```python
from build123d import *

# Parameters (mm, degrees)
F0_W     = 12.5
F0_H     = 7
F1_DEPTH = 8
F2_DEPTH = 2.5


# Not quite as in the source:
# - a feature names something its author has since deleted; it is built from what else it names


with BuildPart() as f1:
    # F0 (on Top) → F1 (new body)
    with BuildSketch(Plane.XY):
        Polygon((-3.75, 44.5469365077), (-3.6919084378, 44.5469365077), (-3.6919084378, 71.5469365077), (-3.6919084378, 78.5469365077), (-8.75, 78.5469365077), (-8.75, 44.5469365077), align=None)
        Polygon((8.75, -44.5469365077), (8.75, 44.5469365077), (3.75, 44.5469365077), (-3.6919084378, 44.5469365077), (-3.75, 44.5469365077), (-8.75, 44.5469365077), (-8.75, -44.5469365077), align=None)
        with BuildLine():
            Line((-4.25, -2.5992627119), (4.25, -2.5992627119))
            Line((4.25, -2.5992627119), (4.25, -17.016687017))
            ThreePointArc((4.25, -17.016687017), (5.7282196187, -19.0992627119), (6.25, -21.5992627119))
            ThreePointArc((6.25, -21.5992627119), (5.7282196187, -24.0992627119), (4.25, -26.1818384069))
            Line((4.25, -26.1818384069), (4.25, -40.5992627119))
            Line((4.25, -40.5992627119), (-4.25, -40.5992627119))
            Line((-4.25, -40.5992627119), (-4.25, -26.1818384069))
            ThreePointArc((-4.25, -26.1818384069), (-6.25, -21.5992627119), (-4.25, -17.016687017))
            Line((-4.25, -17.016687017), (-4.25, -2.5992627119))
        make_face(mode=Mode.SUBTRACT)
        with Locations((2.5580915622, 75.0469365077)):
            Rectangle(F0_W, F0_H)
    extrude(amount=F1_DEPTH)

    # F0 (on Top) → F2 (join)
    with BuildSketch(Plane.XY):
        with BuildLine():
            Line((4.25, -40.5992627119), (4.25, -26.1818384069))
            ThreePointArc((4.25, -26.1818384069), (0, -27.8492627119), (-4.25, -26.1818384069))
            Line((-4.25, -26.1818384069), (-4.25, -40.5992627119))
            Line((-4.25, -40.5992627119), (4.25, -40.5992627119))
        make_face()
        with BuildLine():
            Line((4.25, -26.1818384069), (4.25, -17.016687017))
            ThreePointArc((4.25, -17.016687017), (0, -15.3492627119), (-4.25, -17.016687017))
            Line((-4.25, -17.016687017), (-4.25, -26.1818384069))
            ThreePointArc((-4.25, -26.1818384069), (0, -27.8492627119), (4.25, -26.1818384069))
        make_face()
        with BuildLine():
            Line((4.25, -17.016687017), (4.25, -2.5992627119))
            Line((4.25, -2.5992627119), (-4.25, -2.5992627119))
            Line((-4.25, -2.5992627119), (-4.25, -17.016687017))
            ThreePointArc((-4.25, -17.016687017), (0, -15.3492627119), (4.25, -17.016687017))
        make_face()
        with BuildLine():
            ThreePointArc((6.25, -21.5992627119), (5.7282196187, -19.0992627119), (4.25, -17.016687017))
            Line((4.25, -17.016687017), (4.25, -26.1818384069))
            ThreePointArc((4.25, -26.1818384069), (5.7282196187, -24.0992627119), (6.25, -21.5992627119))
        make_face()
        with BuildLine():
            Line((-4.25, -26.1818384069), (-4.25, -17.016687017))
            ThreePointArc((-4.25, -17.016687017), (-6.25, -21.5992627119), (-4.25, -26.1818384069))
        make_face()
    extrude(amount=F2_DEPTH)


solid = f1.part
```
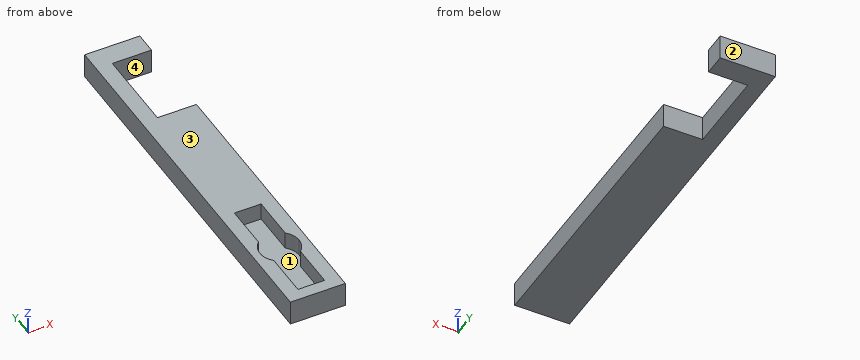
Could you check a few things on this model? Use its own coordinates, in mm. Face numbers are marked on the shaded views. A direction names the side the tool comes from. Round coordinates to 2 decimals unless told otherwise and drop trailing zeros. Loops run counter-clockwise (first coordinate to the right, second up) from the corner with the lowest first, then second, coordinate; pieces in that order, holes last. Notation, with made-up numbers: (-37.5, -1.75) -> (-15.5, -1.75) arc R12 ccw to (-15.5, 15.25) -> close; hole circle Ø10 at (-18.75, 39). An arc over 180 degrees is marked (long way). Put each result on its own line as item: value.
Q1. Which directions (+Z, -Z, +X, -X, +Y, -Y) give clear straight access to the entire face, cutting with the end or side of a thin tool? Please do the marked faces 3 and 4.
Checks:
face 3: +Z, +X, -X, +Y, -Y
face 4: +Z, -Z, +X
Q2. I want a section at C-C on y = -4. Write out the boundary of the cut face in (x, z), and give its area (4 significant figures).
Checks:
outline: (-8.75, 0) -> (8.75, 0) -> (8.75, 8) -> (4.25, 8) -> (4.25, 2.5) -> (-4.25, 2.5) -> (-4.25, 8) -> (-8.75, 8) -> close
area: 93.25 mm2
Q3. For pin 1 Ø4 at (x, y) = (-3.5, -17.5) entering from -Z; pin 2 Ø1.6 at (y, z) = (-34, 4) entering from +X, each with a flat end and sliding along its axis, tell me the tip position at first contact or that it passes through.
Checks:
pin 1: z = 0
pin 2: x = 8.75
Q4. I want a section at A-A on x = 2.5. Write out the boundary of the cut face in (y, z), and give its area (3 significant figures).
Checks:
outline: (-44.55, 0) -> (44.55, 0) -> (44.55, 8) -> (-2.6, 8) -> (-2.6, 2.5) -> (-40.6, 2.5) -> (-40.6, 8) -> (-44.55, 8) -> close; (71.55, 0) -> (78.55, 0) -> (78.55, 8) -> (71.55, 8) -> close
area: 560 mm2
Q5. Please list where these lines run through material, in increasing order: line 1 (Y direction, x = 2.5, z = 5.25); line 2 (Y direction, x = 8.25, z = 1.75); line 3 (X direction, y = -11.5, z = 2.75). Write a range as from..to.
Checks:
line 1: -44.55..-40.6, -2.6..44.55, 71.55..78.55
line 2: -44.55..44.55, 71.55..78.55
line 3: -8.75..-4.25, 4.25..8.75
Q6. Thinking about a two-plate mould opening in X: for the marked faces 1 and 2, which applies, pulls with the +X half, pulls with the -X half, needs draft (parallel to the pull), parting line crosses it, or undercut?
Checks:
face 1: undercut
face 2: needs draft
Q7. I want a section at B-B on z = 5. Write out the boundary of the cut face in (x, y), and give its area (3 significant figures).
Checks:
outline: (-8.75, -44.55) -> (8.75, -44.55) -> (8.75, 44.55) -> (-3.69, 44.55) -> (-3.69, 71.55) -> (8.81, 71.55) -> (8.81, 78.55) -> (-8.75, 78.55) -> close; hole (-4.25, -40.6) -> (4.25, -40.6) -> (4.25, -26.18) arc R6.25 ccw to (4.25, -17.02) -> (4.25, -2.6) -> (-4.25, -2.6) -> (-4.25, -17.02) arc R6.25 ccw to (-4.25, -26.18) -> close
area: 1,470 mm2
